from build123d import *

# Parameters (mm, degrees)
SKETCH_1_W      = 150
SKETCH_1_H      = 100
SKETCH_1_R      = 1.65
SKETCH_1_R_2    = 48.5
EXTRUDE_1_DEPTH = 7.7


with BuildPart() as part:
    # 草图1 → 凸台-拉伸1 (new body)
    with BuildSketch(Plane.XY):
        Rectangle(SKETCH_1_W, SKETCH_1_H)
        with Locations(Location((-65, 30, 0), (0, 0, 180))):
            Circle(SKETCH_1_R, mode=Mode.SUBTRACT)
        with Locations(Location((-65, 10, 0), (0, 0, 180))):
            Circle(SKETCH_1_R, mode=Mode.SUBTRACT)
        with Locations(Location((-65, -10, 0), (0, 0, 180))):
            Circle(SKETCH_1_R, mode=Mode.SUBTRACT)
        with Locations(Location((-65, -30, 0), (0, 0, 180))):
            Circle(SKETCH_1_R, mode=Mode.SUBTRACT)
        with Locations(Location((65, -30, 0), (0, 0, 180))):
            Circle(SKETCH_1_R, mode=Mode.SUBTRACT)
        with Locations(Location((65, -10, 0), (0, 0, 180))):
            Circle(SKETCH_1_R, mode=Mode.SUBTRACT)
        with Locations(Location((65, 10, 0), (0, 0, 180))):
            Circle(SKETCH_1_R, mode=Mode.SUBTRACT)
        with Locations(Location((65, 30, 0), (0, 0, 180))):
            Circle(SKETCH_1_R, mode=Mode.SUBTRACT)
        with Locations(Location((0, 0, 0), (0, 0, 180))):
            Circle(SKETCH_1_R_2, mode=Mode.SUBTRACT)
    extrude(amount=EXTRUDE_1_DEPTH)


solid = part.part
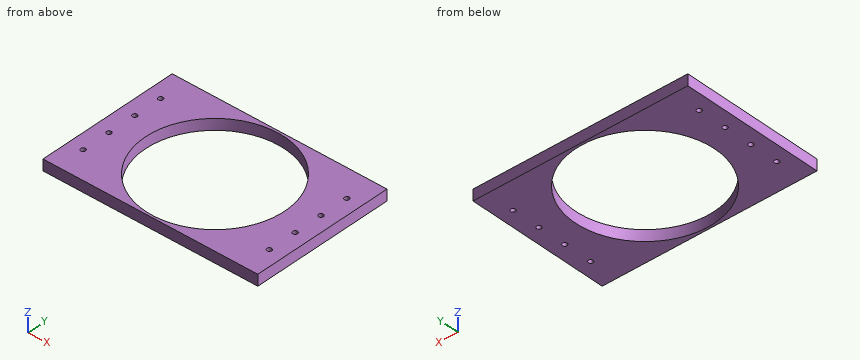
For this review, take the finished solid that the model builds, in its own axes (mm). Round coordinates to 2 decimals unless told otherwise and drop trailing zeros. Loops run counter-clockwise (first coordinate to the right, second up) from the corner with the lowest first, then second, coordinate; pieces in that order, holes last. Notation, with made-up numbers: (-21, 44) - (32, 44) arc R23 cw to (32, 57) - close; hole circle Ø5 at (13, 83). An arc over 180 degrees is marked (long way). One line per item, written item: value. Start each with the question number.
Item 1: Take a section at A-A (y = 0). Give the boundary of the cut face in (x, z), plus the area to 3 significant figures.
Item 2: Take a section at D-D (z = 2.25). State how many separate pieces and enclosed holes the cut face has, plus the area to 3 significant figures.
Item 3: Take a section at C-C (x = 0). Give the boundary of the cut face in (y, z), plus the area to 3 significant figures.
Item 4: Take a section at B-B (x = -65). Give the boundary of the cut face in (y, z).
Item 5: For L1, parallel to Y at x = -65, z = 5; L2, parallel to X at y = 10, z = 3.75; L3, parallel to X at y = -30, z = 6, list the stretches that pass through material, from the lowest coordinate up.
Item 6: Clearance check with a flat-ended pin moving along its axis: pin 1 Ø3 at (x, y) = (65, -30) entering from +Z. State where the tip first meets the part, or that it passes through.
Answer below:
1. outline: (-75, 0) - (-48.5, 0) - (-48.5, 7.7) - (-75, 7.7) - close; (48.5, 0) - (75, 0) - (75, 7.7) - (48.5, 7.7) - close
1. area: 408 mm2
2. separate pieces: 1
2. enclosed holes: 9
2. area: 7,540 mm2
3. outline: (-50, 0) - (-48.5, 0) - (-48.5, 7.7) - (-50, 7.7) - close; (48.5, 0) - (50, 0) - (50, 7.7) - (48.5, 7.7) - close
3. area: 23.1 mm2
4. outline: (-50, 0) - (-31.65, 0) - (-31.65, 7.7) - (-50, 7.7) - close; (-28.35, 0) - (-11.65, 0) - (-11.65, 7.7) - (-28.35, 7.7) - close; (-8.35, 0) - (8.35, 0) - (8.35, 7.7) - (-8.35, 7.7) - close; (11.65, 0) - (28.35, 0) - (28.35, 7.7) - (11.65, 7.7) - close; (31.65, 0) - (50, 0) - (50, 7.7) - (31.65, 7.7) - close
5. L1: y = -50 to -31.65, -28.35 to -11.65, -8.35 to 8.35, 11.65 to 28.35, 31.65 to 50
5. L2: x = -75 to -66.65, -63.35 to -47.46, 47.46 to 63.35, 66.65 to 75
5. L3: x = -75 to -66.65, -63.35 to -38.11, 38.11 to 63.35, 66.65 to 75
6. pin 1: passes through
